The listing builds one solid part. Answer for the finished solid, in the listing's coordinates (mm). Give positions to 0.01 mm unless a question says otherwise; leave off trailing zeros. Loops run counter-clockwise (first coordinate to the right, second up) from the corner with the lowest first, then second, coordinate; pieces in that order, holes last. Notation, with made-up numbers: (67, -34) - (90, -34) arc R6 cw to (90, -25) - close; hole circle Ø5 at (29, 0). An arc over 180 degrees is marked (long way). Answer as CSV lines item,"result". Start each with the question number.
1) A cutting plane is placed at C-C (y = 2.8). Determine the outline of the cut face in (x, z).
2) For a pull along Z with two mould halves and no side action, classify faces 1 (the face through (6.465, 2.154, -3.802)), 2 (the face through (-2, 5, -5)), 3 (the face through (6.526, 2.154, 3.698)), 4 (the face through (1.08, 2.46, 4.88)) as pulls with the +Z half, pulls with the -Z half, needs draft (parallel to the pull), parting line crosses it, or undercut.
3) Find the intervals of material crossed by line 1 along Z through (x, y) = (0, 2.35); line 2 along Z through (x, y) = (-3.25, 2.6); line 3 along Y through (x, z) = (-1, 5.75), in increasing order.
4) A flat-ended cylindrical pin translates along its axis: pin 1 (2 mm diameter, centred on x = -6, y = 3.5, fed in from +Z). Find the tip coordinate at first contact, or state that the pin passes through.
5) A cutting plane is placed at B-B (y = 1.45). Determine the outline of the cut face in (x, z).
6) A cutting plane is placed at A-A (x = 0). Determine the outline of the cut face in (y, z), and give its area (3 significant figures).
Autodesk Inventor part; units mm, degrees
ref_plane "YZ Plane" through (0, 0, 0) normal (1, 0, 0) x (0, 1, 0)
ref_plane "XZ Plane" through (0, 0, 0) normal (0, 1, 0) x (-1, 0, 0)
ref_plane "XY Plane" through (0, 0, 0) normal (0, 0, 1) x (1, 0, 0)
sketch "Sketch1" plane through (0, 0, 0) normal (0, 1, 0) x (-1, 0, 0)
  line L0 (-8.6603, 0) -> (-4.3301, 7.5)
  line L1 (-4.3301, 7.5) -> (4.3301, 7.5)
  line L2 (4.3301, 7.5) -> (8.6603, 0)
  line L3 (8.6603, 0) -> (4.3301, -7.5)
  line L4 (4.3301, -7.5) -> (-4.3301, -7.5)
  line L5 (-4.3301, -7.5) -> (-8.6603, 0)
  circle A0 centre (0, 0) radius 5
  dimension "d0" = 15
  dimension "d1" = 10
extrude "Extrusion1" add sketch "Sketch1" along normal blind 5
sketch "Sketch5" plane through (0, 0, 0) normal (0, 0, 1) x (1, 0, 0)
  line L0 (8.6603, 5) -> (4.3301, 5)
  line L1 (5.6603, 5) -> (8.6603, 5)
  line L2 (8.6603, 2) -> (8.6603, 2.1818)
  arc A0 (8.6603, 2) -> (5.6603, 5) centre (5.6603, 2) ccw
  line L3 (8.6603, 2) -> (8.6603, 5)
  line L4 (0, 0) -> (0, 10.7408) construction
  dimension "d6" = 3
revolve "Revolution1" cut sketch "Sketch5" angle 360 about axis through (0, 0, 0) along (0, 1, 0)
thread "Thread1"
properties part number "NUT"
Ans:
1,outline,"(-8.55, -0.19) - (-4.44, -7.31) arc R8.55 ccw to (-4.11, -7.5) - (4.11, -7.5) arc R8.55 ccw to (4.44, -7.31) - (8.55, -0.19) arc R8.55 ccw to (8.55, 0.19) - (4.44, 7.31) arc R8.55 ccw to (4.11, 7.5) - (-4.11, 7.5) arc R8.55 ccw to (-4.44, 7.31) - (-8.55, 0.19) arc R8.55 ccw to start; hole circle Ø10 at (0, 0)"
2,face 1,"pulls with the -Z half"
2,face 2,"needs draft"
2,face 3,"pulls with the +Z half"
2,face 4,"undercut"
3,line 1,"-7.5 to -5, 5 to 7.5"
3,line 2,"-7.5 to -3.8, 3.8 to 7.5"
3,line 3,"0 to 4.99"
4,pin 1,"z = 6.34"
5,outline,"(-8.66, 0) - (-4.33, -7.5) - (4.33, -7.5) - (8.66, 0) - (4.33, 7.5) - (-4.33, 7.5) - close; hole circle Ø10 at (0, 0)"
6,outline,"(0, -7.5) - (4.37, -7.5) arc R3 ccw to (5, -5.66) - (5, -5) - (0, -5) - close; (0, 5) - (5, 5) - (5, 5.66) arc R3 ccw to (4.37, 7.5) - (0, 7.5) - close"
6,area,"24.3 mm2"
